Geometry check sheet. Reference: the model listing, model coordinates, mm. Face numbers are marked on the shaded views. Coordinates: 2 decimals unless noted, no trailing zeros. Order: outer loops, then holes, each group sorted by start corner. A loop starts at its lowest first (then second) coordinate and runs counter-clockwise, first axis right, second up. Notation, with made-up numbers: (15, 8.5) - (31, 8.5) arc R10 cw to (31, 12.5) - close; hole circle Ø10 at (75, 81). An arc over 180 degrees is marked (long way). Return JSON: item names as keys, results as strings. Group by question number.
Item 1: Section check A-A on x = 0. Enter the section's corners in (y, z).
Item 2: Scan lines: probe 1 along Z at (x, y) = (0, -32); probe 2 along Z at (x, y) = (-2.5, -47); probe 3 along Z at (x, y) = (-19, -15.5). Record each from-to range of solid material in increasing order.
Item 3: Draft check along Z on the marked faces 1, 2 and 3. Enter one of: pulls with the +Z half, pulls with the -Z half, needs draft (parallel to the pull), parting line crosses it, or undercut.
Item 4: Gauge pin test, flat ends, axial feed: pin 1 (4 mm diameter, centred on x = 9, y = -37.5, fed in from -Z); pin 2 (1.5 mm diameter, centred on x = -5, y = -27.5, fed in from -Z); pin 3 (1.5 mm diameter, centred on x = 20, z = 13.5, fed in from +Y). Record the tip position at first contact, or that the pin passes through.
Item 5: Section check B-B on y = -46.5. Give the number of separate pieces and of enclosed holes in the cut face, then the cut area to 3 significant figures.
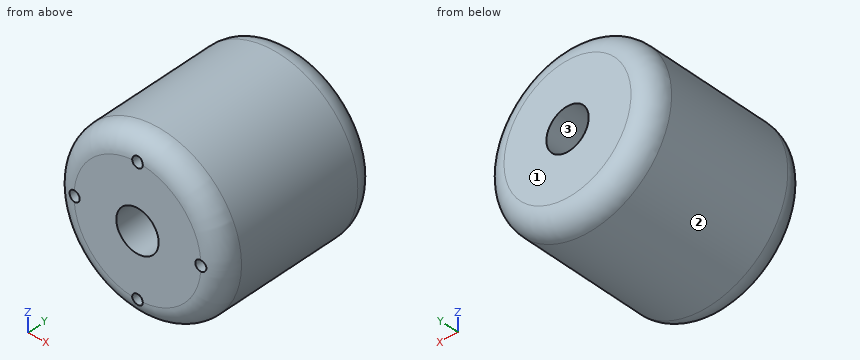
from build123d import *

# Parameters (mm, degrees)
F0_R     = 25.4
F1_DEPTH = 50.8
F2_R     = 6.35
F3_DEPTH = 50.8
F4_R     = 1.5875
F5_DEPTH = 44.45
F7_R     = 6.35


# Not quite as in the source:
# - a fillet or chamfer that OpenCascade refuses, or shapes differently, is made with other operations: its cross-section is extruded or revolved along the edge and cut away or added


with BuildPart() as f1:
    # F0 (on Front) → F1 (new body)
    with BuildSketch(Plane.XZ):
        Circle(F0_R)
    extrude(amount=F1_DEPTH)

    # F2 (on face) → F3 (cut)
    with BuildSketch(Plane.XZ.offset(50.8)):
        Circle(F2_R)
    extrude(amount=-F3_DEPTH, mode=Mode.SUBTRACT)

    # F4 (on face) → F5 (cut)
    with BuildSketch(Plane.XZ.offset(50.8)):
        with Locations((0, 19.0319661051)):
            Circle(F4_R)
        with Locations((18.9372766763, 0)):
            Circle(F4_R)
        with Locations((0, -19.0319661051)):
            Circle(F4_R)
        with Locations((-18.9372785389, 0)):
            Circle(F4_R)
    extrude(amount=-F5_DEPTH, mode=Mode.SUBTRACT)

    # F6: fillet of radius 6.35 on 1 edges, made by hand

    # F6_s1 → F6_t2 (revolve, cut)
    with BuildSketch(Plane.XY):
        with BuildLine():
            ThreePointArc((25.4, -44.45), (23.5401280605, -48.9401280605), (19.05, -50.8))
            Line((19.05, -50.8), (25.4, -50.8))
            Line((25.4, -50.8), (25.4, -44.45))
        make_face()
    revolve(axis=Axis((0, -50.8, 0), (0, -1, 0)), mode=Mode.SUBTRACT)

    # F7
    f7_edges = [f1.edges().sort_by_distance(p)[0] for p in [
        (-25.4, 0, 0),
    ]]
    fillet(f7_edges, radius=F7_R)


solid = f1.part
Computed:
{
 "1": {"outline": "(-50.8, -17.44) - (-6.35, -17.44) - (-6.35, -20.62) - (-50.6, -20.62) arc R6.35 ccw to (-44.45, -25.4) - (-6.35, -25.4) arc R6.35 ccw to (0, -19.05) - (0, -6.35) - (-50.8, -6.35) - close; (-50.8, 6.35) - (0, 6.35) - (0, 19.05) arc R6.35 ccw to (-6.35, 25.4) - (-44.45, 25.4) arc R6.35 ccw to (-50.6, 20.62) - (-6.35, 20.62) - (-6.35, 17.44) - (-50.8, 17.44) - close"},
 "2": {"probe 1": "z = -25.4 to -20.62, -17.44 to -6.35, 6.35 to 17.44, 20.62 to 25.4", "probe 2": "z = -24.74 to -5.84, 5.84 to 24.74", "probe 3": "z = -16.86 to -1.59, 1.59 to 16.86"},
 "3": {"face 1": "needs draft", "face 2": "parting line crosses it", "face 3": "undercut"},
 "4": {"pin 1": "stops at z = -24.42", "pin 2": "stops at z = -25.04", "pin 3": "stops at y = -1.71"},
 "5": {"separate pieces": "1", "enclosed holes": "5", "area": "1,810 mm²"}
}
